The listing builds one solid part. Answer for the finished solid, in the listing's coordinates (mm). Face numbers are marked on the shaded views. A direction names the side the tool comes from. Give positions to 0.01 mm unless a question says otherwise; leave off trailing zeros. Loops run counter-clockwise (first coordinate to the right, second up) from the corner with the lowest first, then second, coordinate; pieces in that order, holes last. Notation, with made-up numbers: (-39.75, 6) - (-27.75, 6) arc R27 ccw to (-27.75, 23) - close; hole circle Ø3 at (35, 53.25). An arc over 180 degrees is marked (long way). Write each question's results on one line, items separated by ' | '.
from build123d import *

# Parameters (mm, degrees)
F0_R          = 9
F0_R_2        = 8
F1_DEPTH      = 5
F2_DEPTH      = 11
F3_R          = 2.5
F4_DEPTH      = 0.5
F5_R          = 1.5
F6_DEPTH      = 25
F5_R_2        = 1
F7_DEPTH      = 8
F8_R          = 1.5
F9_DEPTH      = 9.001
F9_DEPTH_BACK = 9.001


with BuildPart() as f1:
    # F0 (on Front) → F1 (new body)
    with BuildSketch(Plane.XZ):
        Circle(F0_R)
        Circle(F0_R_2, mode=Mode.SUBTRACT)
        Circle(F0_R_2)
    extrude(amount=F1_DEPTH)

    # F0 (on Front) → F2 (join)
    with BuildSketch(Plane.XZ):
        Circle(F0_R_2)
    extrude(amount=-F2_DEPTH)

    # F3 (on face) → F4 (join)
    with BuildSketch(Plane(origin=(0, 11, 0), x_dir=(-1, 0, 0), z_dir=(0, 1, 0))):
        Circle(F3_R)
    extrude(amount=F4_DEPTH)

    # F5 (on face) → F6 (cut)
    with BuildSketch(Plane.XZ.offset(5)):
        Circle(F5_R)
    extrude(amount=-F6_DEPTH, mode=Mode.SUBTRACT)

    # F5 (on face) → F7 (join)
    with BuildSketch(Plane.XZ.offset(5)):
        with Locations((0, 4)):
            Circle(F5_R_2)
    extrude(amount=F7_DEPTH)

    # F8 (on Right) → F9 (cut, two sides)
    with BuildSketch(Plane.YZ) as f9_sk:
        with Locations((7, 0)):
            Circle(F8_R)
    extrude(amount=-F9_DEPTH, mode=Mode.SUBTRACT)
    extrude(f9_sk.sketch, amount=F9_DEPTH_BACK, mode=Mode.SUBTRACT)


solid = f1.part
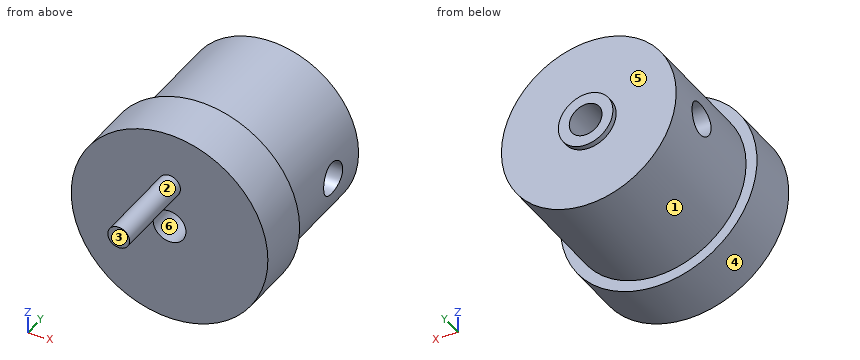
Item 1: Find the intervals of material crossed by line 1 along Z through (x, y) = (0, 10.55); line 2 along Y through (x, z) = (6.5, 5.5), in increasing order. Write a range as [from, to].
Values found:
line 1: z = [-8, -1.5], [1.5, 8] | line 2: y = [-5, 0]
Item 2: Flat-ended cylindrical pins translate along their axes: P1, Ø6, axis at x = 3.5, z = -5, coming from the -Y side; P2, Ø8, axis at y = 2.5, z = 7, coming from the +X side; P3, Ø1.5, axis at x = -7, y = 8.5, coming from the -Z side; P4, Ø6, axis at y = -2.5, z = 2.5, coming from the -X side. Find the tip coordinate at first contact, or state that the pin passes through.
Values found:
P1: stops at y = -5 | P2: stops at x = 8.12 | P3: stops at z = -4.99 | P4: stops at x = -9
Item 3: A cutting plane is placed at A-A, the plane y = 7.75. Determine the outline of the cut face in (x, z), plus the area to 3 significant figures.
Values found:
outline: (-7.89, -1.3) arc R8 ccw to (7.89, -1.3) - (0.75, -1.3) arc R1.5 cw to (-0.75, -1.3) - close; (-7.89, 1.3) - (-0.75, 1.3) arc R1.5 cw to (0.75, 1.3) - (7.89, 1.3) arc R8 ccw to start | area: 159 mm²
Item 4: For the marked faces 1, 2 and 3, determine the directions among +Z, -Z, +X, -X, +Y, -Y from which every point of the face is accessible in a straight line to the end or side of a thin tool.
Values found:
face 1: +Y | face 2: -Y | face 3: +Z, -Z, +X, -X, -Y
Item 5: A cutting plane is placed at B-B, the plane z = 0. Determine the outline of the cut face in (x, y), plus the area to 3 significant figures.
Values found:
outline: (-9, -5) - (-1.5, -5) - (-1.5, 5.5) - (-8, 5.5) - (-8, 0) - (-9, 0) - close; (-8, 8.5) - (-1.5, 8.5) - (-1.5, 11.5) - (-2.5, 11.5) - (-2.5, 11) - (-8, 11) - close; (1.5, -5) - (9, -5) - (9, 0) - (8, 0) - (8, 5.5) - (1.5, 5.5) - close; (1.5, 8.5) - (8, 8.5) - (8, 11) - (2.5, 11) - (2.5, 11.5) - (1.5, 11.5) - close | area: 180 mm²
Item 6: A cutting plane is placed at D-D, the plane z = 4. Determine the outline of the cut face in (x, y).
Values found:
outline: (-8.06, -5) - (-1, -5) - (-1, -13) - (1, -13) - (1, -5) - (8.06, -5) - (8.06, 0) - (6.93, 0) - (6.93, 11) - (-6.93, 11) - (-6.93, 0) - (-8.06, 0) - close
Item 7: A cutting plane is placed at C-C, the plane x = -4.75. Determine the outline of the cut face in (y, z), plus the area to 3 significant figures.
Values found:
outline: (-5, -7.64) - (0, -7.64) - (0, -6.44) - (11, -6.44) - (11, 6.44) - (0, 6.44) - (0, 7.64) - (-5, 7.64) - close; hole circle Ø3 at (7, 0) | area: 211 mm²
Item 8: For a pull along X with two mould halves and no side action, classify the marked faces 4, 5 and 6 as released by +X, released by -X, zero draft, split by the parting line, or undercut.
Values found:
face 4: split by the parting line | face 5: zero draft | face 6: undercut
